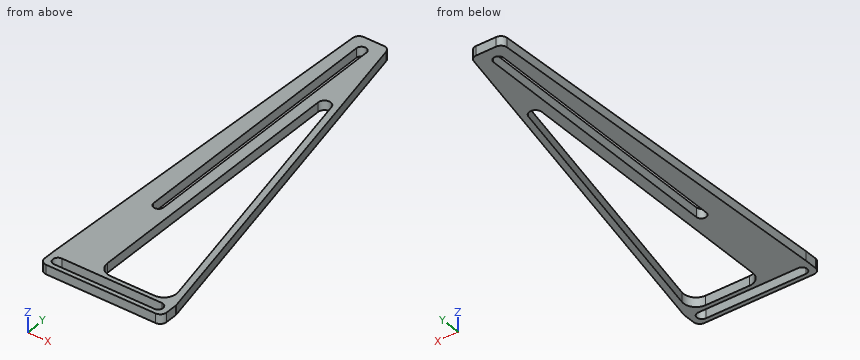
```python
from build123d import *

# Parameters (mm, degrees)
EXTRUDE_1_DEPTH = 3
EXTRUDE_2_DEPTH = 3
FILLET_1_R      = 2
FILLET_2_R      = 4
FILLET_3_R      = 2


with BuildPart() as part:
    # 草图1 → 凸台-拉伸1 (new body)
    with BuildSketch(Plane.XY):
        Polygon((0, 0), (39, 0), (39, 6), (14, 6), (14, 128), (4, 128), (4, 6), (0, 6), align=None)
        with BuildLine():
            Line((3.5, 4.6), (35.5, 4.6))
            ThreePointArc((35.5, 4.6), (37.1, 3), (35.5, 1.4))
            Line((35.5, 1.4), (3.5, 1.4))
            ThreePointArc((3.5, 1.4), (1.9, 3), (3.5, 4.6))
        make_face(mode=Mode.SUBTRACT)
        with BuildLine():
            Line((7.4, 38), (7.4, 123))
            ThreePointArc((7.4, 123), (9, 124.6), (10.6, 123))
            Line((10.6, 123), (10.6, 38))
            ThreePointArc((10.6, 38), (9, 36.4), (7.4, 38))
        make_face(mode=Mode.SUBTRACT)
    extrude(amount=EXTRUDE_1_DEPTH)

    # 草图2 → 凸台-拉伸2 (add)
    with BuildSketch(Plane.XY.offset(3)):
        Polygon((0, 6), (4, 128), (4, 6), align=None)
        Polygon((14, 128), (39, 6), (36.9584404, 6), (14, 118.037189152), align=None)
    extrude(amount=-EXTRUDE_2_DEPTH)

    # 圆角1
    fillet_1_edges = [part.edges().sort_by_distance(p)[0] for p in [
        (0, 6, 1.5),
        (4, 128, 1.5),
        (14, 128, 1.5),
        (39, 6, 1.5),
        (14, 118.037189152, 1.5),
    ]]
    fillet(fillet_1_edges, radius=FILLET_1_R)

    # 圆角2
    fillet_2_edges = [part.edges().sort_by_distance(p)[0] for p in [
        (14, 6, 1.5),
        (36.9584404, 6, 1.5),
    ]]
    fillet(fillet_2_edges, radius=FILLET_2_R)

    # 圆角3
    fillet_3_edges = [part.edges().sort_by_distance(p)[0] for p in [
        (39, 0, 1.5),
        (0, 0, 1.5),
    ]]
    fillet(fillet_3_edges, radius=FILLET_3_R)


solid = part.part
```
The listing builds one solid part. Answer for the finished solid, in the listing's coordinates (mm). Round coordinates to 2 decimals unless told otherwise and drop trailing zeros. Write each loop counter-clockwise with the first axis right and the second up, starting at its lowest first coordinate (ties: lowest second). Pieces come first, ordered by that corner, then holes. Notation, with made-up numbers: (71, 88) -> (89, 88) arc R23 cw to (89, 104) -> close; hole circle Ø8 at (62, 86). An arc over 180 degrees is marked (long way). Write item = value, one per line.
1) Section A-A on x = 9 is taken. Write down the section's boundary in (y, z).
Check values:
outline = (0, 0) -> (1.4, 0) -> (1.4, 3) -> (0, 3) -> close; (4.6, 0) -> (36.4, 0) -> (36.4, 3) -> (4.6, 3) -> close; (124.6, 0) -> (128, 0) -> (128, 3) -> (124.6, 3) -> close
2) Section B-B on z = 1.85 is taken. Write down the section's boundary in (x, y), plus the area to 3 significant figures.
Check values:
outline = (0, 2) arc R2 ccw to (2, 0) -> (37, 0) arc R2 ccw to (39, 2) -> (39, 5.8) arc R2 ccw to (38.96, 6.2) -> (14.33, 126.4) arc R2 ccw to (12.37, 128) -> (5.94, 128) arc R2 ccw to (3.94, 126.07) -> (0, 6) -> close; hole (3.5, 1.4) -> (35.5, 1.4) arc R1.6 ccw to (35.5, 4.6) -> (3.5, 4.6) arc R1.6 ccw to start; hole (7.4, 38) arc R1.6 ccw to (10.6, 38) -> (10.6, 123) arc R1.6 ccw to (7.4, 123) -> close; hole (14, 10) arc R4 ccw to (18, 6) -> (32.06, 6) arc R4 ccw to (35.97, 10.8) -> (17.96, 98.72) arc R2 ccw to (14, 98.31) -> close
area = 1,590 mm²
3) Section D-D on y = 89 is taken. Write down the section's boundary in (x, z).
Check values:
outline = (2.72, 0) -> (7.4, 0) -> (7.4, 3) -> (2.72, 3) -> close; (10.6, 0) -> (14, 0) -> (14, 3) -> (10.6, 3) -> close; (19.95, 0) -> (21.99, 0) -> (21.99, 3) -> (19.95, 3) -> close
4) Given pin 1 (1.5 mm diameter, centred on y = 52, z = 2, fed in from +X); pin 2 (1 mm diameter, centred on y = 38.5, z = 1.5, fed in from -X), each flat-ended and moving along its own axis, determine where each tip first touches the part or whether it passes through.
Check values:
pin_1 = 29.73
pin_2 = 1.05
5) Straight lines are drawn through the part: line 1 along X through (y, z) = (90.5, 1); line 2 along X through (y, z) = (78, 0.35); line 3 along X through (y, z) = (119, 2.4). For each, find the intervals that lie inside material, in ascending order. Write a range as [from, to].
Check values:
line_1 = [2.77, 7.4], [10.6, 14], [19.64, 21.68]
line_2 = [2.36, 7.4], [10.6, 14], [22.2, 24.25]
line_3 = [3.7, 7.4], [10.6, 15.84]
6) Section C-C on y = 110.5 is taken. Write down the section's boundary in (x, z), plus the area to 3 significant figures.
Check values:
outline = (3.43, 0) -> (7.4, 0) -> (7.4, 3) -> (3.43, 3) -> close; (10.6, 0) -> (17.59, 0) -> (17.59, 3) -> (10.6, 3) -> close
area = 32.9 mm²
